Here's how the part is built. I have some questions about the finished solid (model axes, mm). A direction names the side the tool comes from. Give positions to 0.01 mm unless a question says otherwise; leave off trailing zeros. Loops run counter-clockwise (first coordinate to the right, second up) from the corner with the lowest first, then second, coordinate; pieces in that order, holes last. Notation, with made-up numbers: (75.25, 16) - (85.25, 16) arc R17 cw to (85.25, 34) - close; hole circle Ø11 at (52.5, 25.25). An arc over 180 degrees is marked (long way). Return JSON: item names as keys, results as strings. Group by question number.
(1) I need wall thicknesses on probe 1 along Z at (x, y) = (18, -1); probe 2 along Z at (x, y) = (-10, -6); probe 3 along X at (y, z) = (-1, 10.5). Which ranges of each line are inside material? Lowest first, please. Write a range as [from, to].
(2) On a 3-axis mill with a long thin cutter (end or side, diameter ignored), from which of +Z, -Z, +X, -X, +Y, -Y can I reach the whole of each face in a straight line? I mean faces 1 (the flat face through (31.75, -4, 35)), 2 (the flat face through (6.35, -4, 3)), 3 (the flat face through (3, -4, 44.45)). Say none if no direction works.
(3) If we section it at B-B (z = 8): Please give me the cut outline in (x, y).
(4) If we section it at D-D (x = -9.5): Please give me the cut outline in (y, z).
(5) If we mould it in two halves opening along Z, with no side actions, what happens to faces 4 (the flat face through (29, -4, 38.1)), 5 (the flat face through (19.05, -4, 10)), 6 (the flat face through (-19.05, -4, 41))? For each: released by +Z, released by -Z, zero draft, split by the parting line, or undercut.
(6) For P1, Ø1.9, axis at x = 27.5, y = -5.5, coming from the +Z side; P2, Ø1.9, axis at y = -4.5, z = 36, coming from the +X side; P3, Ø1.9, axis at y = -3, z = 40, coming from the -X side, each with a flat end and sliding along its axis, tell me the tip position at first contact or that it passes through.
(7) If we section it at A-A (x = 20): Please give me the cut outline in (y, z).
(8) If we section it at C-C (z = 33.5): Please give me the cut outline in (x, y).
```python
from build123d import *

# Parameters (mm, degrees)
F1_DEPTH = 7.62
F2_W     = 6.35
F2_H     = 6.35
F3_DEPTH = 7.62
F4_R     = 2.54
F5_DEPTH = 7.62


with BuildPart() as f1:
    # F0 (on Front) → F1 (new body)
    with BuildSketch(Plane.XZ):
        Polygon((-19.05, 0), (0, 0), (0, 6.35), (-12.7, 6.35), (-12.7, 12.7), (19.05, 12.7), (19.05, 6.35), (6.35, 6.35), (6.35, 0), (25.4, 0), (25.4, 19.05), (31.75, 19.05), (31.75, 6.35), (38.1, 6.35), (38.1, 31.75), (31.75, 31.75), (31.75, 38.1), (25.4, 38.1), (25.4, 44.45), (19.05, 44.45), (19.05, 50.8), (25.4, 50.8), (25.4, 57.15), (12.7, 57.15), (12.7, 44.45), (-6.35, 44.45), (-6.35, 57.15), (-19.05, 57.15), (-19.05, 50.8), (-12.7, 50.8), (-12.7, 44.45), (-19.05, 44.45), (-19.05, 38.1), (-25.4, 38.1), (-25.4, 31.75), (-31.75, 31.75), (-31.75, 6.35), (-25.4, 6.35), (-25.4, 19.05), (-19.05, 19.05), align=None)
    extrude(amount=F1_DEPTH)

    # F2 (on face) → F3 (cut)
    with BuildSketch(Plane.XZ.offset(7.62)):
        with Locations((-9.525, 34.925)):
            Rectangle(F2_W, F2_H)
        with Locations((15.875, 34.925)):
            Rectangle(F2_W, F2_H)
    extrude(amount=-F3_DEPTH, mode=Mode.SUBTRACT)

    # F4 (on face) → F5 (cut)
    with BuildSketch(Plane.XZ.offset(7.62)):
        with Locations((-9.809578, 53.594287)):
            Circle(F4_R)
    extrude(amount=-F5_DEPTH, mode=Mode.SUBTRACT)


solid = f1.part
```
Values:
{
 "1": {"probe 1": "[0, 6.35], [12.7, 31.75], [38.1, 57.15]", "probe 2": "[0, 6.35], [12.7, 31.75], [38.1, 51.06], [56.13, 57.15]", "probe 3": "[-31.75, -25.4], [-19.05, -12.7], [19.05, 25.4], [31.75, 38.1]"},
 "2": {"face 1": "+Z, +X, +Y, -Y", "face 2": "-Z, +Y, -Y", "face 3": "+Z, +Y, -Y"},
 "3": {"outline": "(-31.75, -7.62) - (-25.4, -7.62) - (-25.4, 0) - (-31.75, 0) - close; (-19.05, -7.62) - (-12.7, -7.62) - (-12.7, 0) - (-19.05, 0) - close; (19.05, -7.62) - (25.4, -7.62) - (25.4, 0) - (19.05, 0) - close; (31.75, -7.62) - (38.1, -7.62) - (38.1, 0) - (31.75, 0) - close"},
 "4": {"outline": "(-7.62, 0) - (0, 0) - (0, 6.35) - (-7.62, 6.35) - close; (-7.62, 12.7) - (0, 12.7) - (0, 31.75) - (-7.62, 31.75) - close; (-7.62, 38.1) - (0, 38.1) - (0, 51.07) - (-7.62, 51.07) - close; (-7.62, 56.12) - (0, 56.12) - (0, 57.15) - (-7.62, 57.15) - close"},
 "5": {"face 4": "released by +Z", "face 5": "undercut", "face 6": "zero draft"},
 "6": {"P1": "z = 38.1", "P2": "x = 31.75", "P3": "x = -19.05"},
 "7": {"outline": "(-7.62, 0) - (0, 0) - (0, 44.45) - (-7.62, 44.45) - close; (-7.62, 50.8) - (0, 50.8) - (0, 57.15) - (-7.62, 57.15) - close"},
 "8": {"outline": "(-25.4, -7.62) - (-12.7, -7.62) - (-12.7, 0) - (-25.4, 0) - close; (-6.35, -7.62) - (12.7, -7.62) - (12.7, 0) - (-6.35, 0) - close; (19.05, -7.62) - (31.75, -7.62) - (31.75, 0) - (19.05, 0) - close"}
}
